For this review, take the finished solid that the model builds, in its own axes (mm). A direction names the side the tool comes from. Give positions to 0.01 mm unless a question says otherwise; leave off trailing zeros. Order: outer loops, then holes, each group sorted by start corner. A loop starts at its lowest first (then second) coordinate and runs counter-clockwise, first axis right, second up. Notation, with made-up numbers: (19.25, -10.75) - (44.25, -10.75) arc R22 ccw to (44.25, 21.25) - close; hole circle Ø1 at (34.25, 35.5). An arc over 180 degrees is marked (long way). One line per item, written item: value.
Autodesk Fusion 360 part; units mm, degrees
sketch "Sketch1" plane through (0, 0, 0) normal (0, 0, 1) x (1, 0, 0)
  line L0 (0, 0) -> (40, 0)
  line L1 (0, 0) -> (5, 8)
  line L2 (35, 8) -> (40, 0)
  line L3 (5, 8) -> (-10, 8)
  line L4 (-10, 8) -> (-10, 20)
  line L5 (-10, 20) -> (50, 20)
  line L6 (50, 20) -> (50, 8)
  line L7 (50, 8) -> (35, 8)
  line L8 (-5, 20) -> (-5, 40)
  line L9 (-5, 40) -> (5, 40)
  line L10 (15, 30) -> (25, 30)
  line L11 (35, 40) -> (45, 40)
  line L12 (45, 40) -> (45, 20)
  line L13 (5, 40) -> (15, 30)
  line L14 (35, 40) -> (25, 30)
  dimension "d1" = 40
  dimension "d2" = 30
  dimension "d5" = 12
  dimension "d8" = 60
  dimension "d9" = 5
  dimension "d10" = 5
  dimension "d11" = 10
  dimension "d14" = 10
  dimension "d15" = 10
  dimension "d16" = 20
  dimension "d17" = 8
extrude "Extrude1" add sketch "Sketch1" against normal blind 50
chamfer "Chamfer1" distance 10 distance2 20 1 edges at (0, 40, 0) measured on face at (-1.6667, 40, -16.6667)
chamfer "Chamfer2" distance 20 distance2 10 1 edges at (40, 40, -50) measured on face at (18.3333, 15.3333, -50)
(1) Take a section at C-C (z = -35). Write out the cut boundary in (x, y).
Answers below:
outline: (-10, 8) - (5, 8) - (0, 0) - (40, 0) - (35, 8) - (50, 8) - (50, 20) - (45, 20) - (45, 40) - (35, 40) - (25, 30) - (15, 30) - (5, 40) - (-5, 40) - (-5, 20) - (-10, 20) - close
(2) For P1, Ø12, axis at x = 18, z = -43.5, coming from the +Y side; P2, Ø8, axis at x = 9.5, y = 35.5, coming from the +Z side; P3, Ø4, axis at x = 47.5, z = -30.5, coming from the +Y side, all flat-tipped, find the tip position at first contact; note any pin that passes through.
Answers below:
P1: stops at y = 33
P2: stops at z = -5.75
P3: stops at y = 20
(3) Machinability: for faces 1 (the face through (-2, 8, -25)), 2 (the face through (-5, 30, -25)), 3 (the face through (43, 8, -25)), 4 (the face through (47, 20, -25)), which of the approach directions +Z, -Z, +X, -X, +Y, -Y give a long, thin tool a straight path to every point of the face, cutting with its end or side? Answer none if there is none.
Answers below:
face 1: +Z, -Z, -X
face 2: +Z, -Z, -X, +Y
face 3: +Z, -Z, +X
face 4: +Z, -Z, +X, +Y
(4) Take a section at D-D (x = 29). Write out the cut boundary in (y, z), then the cut area to 3 significant figures.
Answers below:
outline: (0, -50) - (20, -50) - (34, -43) - (34, -7) - (20, 0) - (0, 0) - close
area: 1,600 mm^2
(5) Take a section at A-A (x = 1.5). Write out the cut boundary in (y, z), then the cut area to 3 significant figures.
Answers below:
outline: (0, -50) - (2.4, -50) - (2.4, 0) - (0, 0) - close; (8, -50) - (20, -50) - (40, -40) - (40, -10) - (20, 0) - (8, 0) - close
area: 1,520 mm^2
(6) Take a section at B-B (y = 38). Write out the cut boundary in (x, z).
Answers below:
outline: (-5, -41) - (7, -41) - (7, -9) - (-5, -9) - close; (33, -41) - (45, -41) - (45, -9) - (33, -9) - close
(7) Wall thickness on line 1 (Y direction, x = 1.5, z = -43.5); line 2 (X direction, y = 21, z = -5.5); line 3 (Y direction, x = 24, z = -2.5): over which ranges is each line inside the solid? List them lowest first. Write a range as from..to.
Answers below:
line 1: y = 0..2.4, 8..33
line 2: x = -5..45
line 3: y = 0..25
(8) Draft analysis for pull direction Y (two halves, no side actions). For faces 5 (the face through (37.465, 4.056, -24.65)), 6 (the face through (20, 12, 0)), 7 (the face through (-8, 20, -25)), state which applies: pulls with the +Y half, pulls with the -Y half, needs draft (parallel to the pull), parting line crosses it, or undercut.
Answers below:
face 5: undercut
face 6: needs draft
face 7: pulls with the +Y half
